```python
from build123d import *

# Parameters (mm, degrees)
F0_R     = 34.925
F1_DEPTH = 20.32
F2_R     = 10.15999
F3_W     = 3.175
F3_H     = 3.175
F4_DEPTH = 20.32


# Not quite as in the source:
# - a fillet or chamfer is up to 0.001 mm smaller than in the source, because OpenCascade refuses the exact size


with BuildPart() as f1:
    # F0 (on Front) → F1 (new body)
    with BuildSketch(Plane.XZ):
        Circle(F0_R)
    extrude(amount=F1_DEPTH)

    # F2 (radius 10.16 in the source; OpenCascade refuses exactly that, so slightly less here)
    f2_edges = [f1.edges().sort_by_distance(p)[0] for p in [
        (-34.925, -20.32, 0),
        (-34.925, 0, 0),
    ]]
    fillet(f2_edges, radius=F2_R)

    # F3 (on face) → F4 (cut, through all)
    with BuildSketch(Plane.XZ.offset(20.32)):
        Rectangle(F3_W, F3_H)
    extrude(amount=-F4_DEPTH, mode=Mode.SUBTRACT)


solid = f1.part
```
Work out the finished part from the listing and answer in its coordinate system (mm). A direction names the side the tool comes from. Give positions to 0.01 mm unless a question says otherwise; leave off trailing zeros. Order: outer loops, then holes, each group sorted by start corner. A loop starts at its lowest first (then second) coordinate and runs counter-clockwise, first axis right, second up. Notation, with made-up numbers: (87.25, -27) - (132.25, -27) arc R21 cw to (132.25, -13) - close; hole circle Ø7 at (58.5, -23). An arc over 180 degrees is marked (long way). One line per item, written item: value. Start each with the question number.
1. Consider line 1 (X direction, y = -9.25, z = -3); line 2 (Z direction, x = -19, y = -1.5); line 3 (X direction, y = -17.25, z = -3.5). Determine where each line is inside the solid, lowest interval first.
2. Which of the six approach directions +Z, -Z, +X, -X, +Y, -Y give full straight-line access (tool end or side, diameter ignored) to faces 3 (the face through (0, -20.32, -5)), 4 (the face through (0, -10, 1.588))?
3. Each of these flat-tipped pins is pushed along its axis until it touches: pin 1 Ø2 at (y, z) = (-17.5, 18.5) entering from +X; pin 2 Ø1.5 at (y, z) = (-6.5, -15) entering from +X; pin 3 Ø2 at (x, y) = (18.5, -6.5) entering from +Z. Where does it stop, or does it pass through?
4. Section D-D, the plane y = -5.5 is taken. Write down the section's boundary in (x, z).
5. For a pull along X with two mould halves and no side action, classify faces 1 (the face through (0, 0, -5)), 2 (the face through (1.588, -10, 0)) as released by +X, released by -X, zero draft, split by the parting line, or undercut.
6. Section C-C, the plane y = -18.5 is taken. Write down the section's boundary in (x, z).
Filled sheet:
1. line 1: -34.75 to 34.75
1. line 2: -23.32 to 23.32
1. line 3: -31.85 to 31.85
2. face 3: +Z, -Z, +X, -X, -Y
2. face 4: +Y, -Y
3. pin 1: x = 27.18
3. pin 2: x = 31.25
3. pin 3: z = 29.56
4. outline: circle Ø67.59 at (0, 0); hole (-1.59, -1.59) - (1.59, -1.59) - (1.59, 1.59) - (-1.59, 1.59) - close
5. face 1: zero draft
5. face 2: undercut
6. outline: circle Ø61.14 at (0, 0); hole (-1.59, -1.59) - (1.59, -1.59) - (1.59, 1.59) - (-1.59, 1.59) - close
